Design review of the part built by this model. Coordinates are the model's own, in mm. A direction names the side the tool comes from. Give positions to 0.01 mm unless a question says otherwise; leave off trailing zeros. Order: outer loops, then holes, each group sorted by start corner. A loop starts at its lowest first (then second) coordinate and runs counter-clockwise, first axis right, second up.
```python
from build123d import *

# Parameters (mm, degrees)
SKETCH_R        = 1.8
PAD_DEPTH       = 3.8
SKETCH001_R     = 1.8
POCKET_DEPTH    = 5
SKETCH002_W     = 2
SKETCH002_H     = 10
PAD001_DEPTH    = 5
SKETCH003_R     = 2
POCKET001_DEPTH = 5


with BuildPart() as part:
    # Sketch → Pad (new body)
    with BuildSketch(Plane.XY):
        Polygon((0, 0), (0, 20), (18, 20), (18, 30), (52, 30), (52, 20), (70, 20), (70, 0), (52, 0), (52, -10), (18, -10), (18, 0), align=None)
        with Locations((27.5, 25)):
            Circle(SKETCH_R, mode=Mode.SUBTRACT)
        with Locations((42.5, 25)):
            Circle(SKETCH_R, mode=Mode.SUBTRACT)
        with Locations((27.5, -5)):
            Circle(SKETCH_R, mode=Mode.SUBTRACT)
        with Locations((42.5, -5)):
            Circle(SKETCH_R, mode=Mode.SUBTRACT)
    extrude(amount=PAD_DEPTH)

    # Sketch001 → Pocket (cut)
    with BuildSketch(Plane.XY.offset(3.8)):
        with Locations((5, 15)):
            Circle(SKETCH001_R)
        with Locations((65, 15)):
            Circle(SKETCH001_R)
        with Locations((65, 5)):
            Circle(SKETCH001_R)
        with Locations((5, 5)):
            Circle(SKETCH001_R)
    extrude(amount=-POCKET_DEPTH, mode=Mode.SUBTRACT)

    # Sketch002 → Pad001 (new body)
    with BuildSketch(Plane.XY.offset(3.8)):
        with Locations((19, 25)):
            Rectangle(SKETCH002_W, SKETCH002_H)
        with Locations((51, 25)):
            Rectangle(SKETCH002_W, SKETCH002_H)
        with Locations((51, -5)):
            Rectangle(SKETCH002_W, SKETCH002_H)
        with Locations((19, -5)):
            Rectangle(SKETCH002_W, SKETCH002_H)
    extrude(amount=PAD001_DEPTH)

    # Sketch003 → Pocket001 (cut)
    with BuildSketch(Plane.XY.offset(3.8)):
        with Locations((10, 10)):
            Circle(SKETCH003_R)
        with Locations((20, 10)):
            Circle(SKETCH003_R)
        with Locations((30, 10)):
            Circle(SKETCH003_R)
        with Locations((40, 10)):
            Circle(SKETCH003_R)
        with Locations((50, 10)):
            Circle(SKETCH003_R)
        with Locations((60, 10)):
            Circle(SKETCH003_R)
    extrude(amount=-POCKET001_DEPTH, mode=Mode.SUBTRACT)


solid = part.part
```
1. Take a section at C-C (y = -5). State the section outline as (x, z) points.
Recorded:
outline: (18, 0) - (25.7, 0) - (25.7, 3.8) - (20, 3.8) - (20, 8.8) - (18, 8.8) - close; (29.3, 0) - (40.7, 0) - (40.7, 3.8) - (29.3, 3.8) - close; (44.3, 0) - (52, 0) - (52, 8.8) - (50, 8.8) - (50, 3.8) - (44.3, 3.8) - close
2. For pin 1 (2 mm diameter, centred on x = 55, z = 2.5, fed in from +Y); pin 2 (2.5 mm diameter, centred on x = 30, y = 10, fed in from -Z); pin 3 (20 mm diameter, centred on x = 39, y = 18, fed in from +Z); pin 4 (8 mm diameter, centred on x = 10.5, y = 22.5, fed in from -Z), all flat-tipped, find the tip position at first contact; note any pin that passes through.
Recorded:
pin 1: stops at y = 20
pin 2: passes through
pin 3: stops at z = 3.8
pin 4: stops at z = 0
3. Machinability: for faces 4 (the face through (0, 10, 2)), 5 (the face through (51.908, 10.601, 1.927)), 6 (the face through (20, 25, 6)), 7 (the face through (18, 25, 4)), 8 (the face through (9, 0, 2)), which of the approach directions +Z, -Z, +X, -X, +Y, -Y give a long, thin tool a straight path to every point of the face, cutting with its end or side? Answer none if there is none.
Recorded:
face 4: +Z, -Z, -X, +Y, -Y
face 5: +Z, -Z
face 6: +Z, +Y, -Y
face 7: +Z, -Z, -X, +Y
face 8: +Z, -Z, -X, -Y
4. Take a section at B-B (z = 6). State the section outline as (x, y) points, then the cut area to 3 significant figures.
Recorded:
outline: (18, -10) - (20, -10) - (20, 0) - (18, 0) - close; (18, 20) - (20, 20) - (20, 30) - (18, 30) - close; (50, -10) - (52, -10) - (52, 0) - (50, 0) - close; (50, 20) - (52, 20) - (52, 30) - (50, 30) - close
area: 80.0 mm2
5. For line 1 along Y through (x, z) = (27.5, 1.9); line 2 along X through (y, z) = (-6, 6.5); line 3 along Y through (x, z) = (65, 1.4), list the stretches that pass through material, from the lowest coordinate up.
Recorded:
line 1: y = -10 to -6.8, -3.2 to 23.2, 26.8 to 30
line 2: x = 18 to 20, 50 to 52
line 3: y = 0 to 3.2, 6.8 to 13.2, 16.8 to 20
6. Draft analysis for pull direction Y (two halves, no side actions). For faces 1 (the face through (51, 20, 6)), 2 (the face through (52, 25, 4)), 3 (the face through (35, -10, 2)), state which applies: pulls with the +Y half, pulls with the -Y half, needs draft (parallel to the pull), parting line crosses it, or undercut.
Recorded:
face 1: undercut
face 2: needs draft
face 3: pulls with the -Y half
7. Take a section at A-A (x = 10). State the section outline as (y, z) points.
Recorded:
outline: (0, 0) - (8, 0) - (8, 3.8) - (0, 3.8) - close; (12, 0) - (20, 0) - (20, 3.8) - (12, 3.8) - close
8. Take a section at D-D (z = 1). State how many separate pieces and enclosed holes the cut face has, then the cut area to 3 significant figures.
Recorded:
separate pieces: 1
enclosed holes: 14
area: 1,920 mm2
